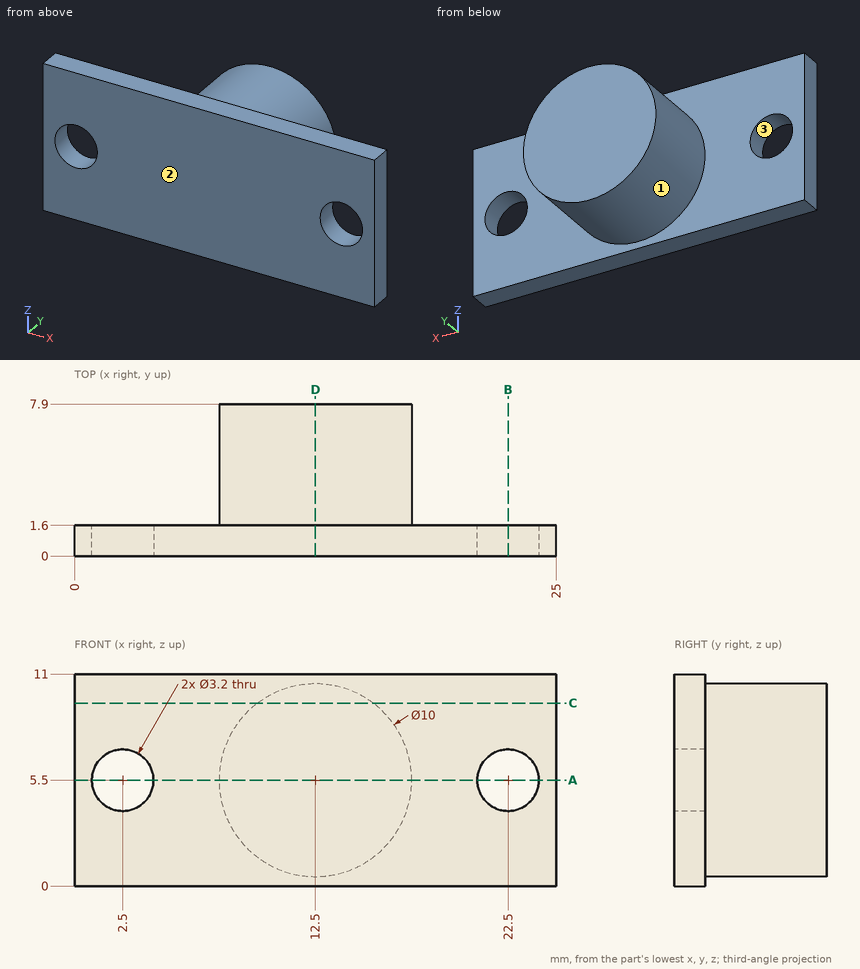
Drawing for the job (mm, zero at the part's lowest x, y, z). Give positions to 0.01 mm unless a question says otherwise; leave off trailing zeros. Order: outer loops, then holes, each group sorted by start corner. A loop starts at its lowest first (then second) coordinate and runs counter-clockwise, first axis right, second up. Notation, with made-up numbers: M 5.5,59 L 33.5,59 A7 ccw 33.5,65 Z; hole C 86.5,79.5 d6. An arc over 180 degrees is marked long. Put each result on its own line as item: value. Start each with the question number.
(1) Saw through at B-B, the plane x = 22.5. Write the cut outline in (y, z), then the cut area to 3 significant figures.
(2) Mould opens along X. For the marked faces 1, 2 and 3 say: +X half, -X half, draft (parallel to the pull), parting line (faces both ways), or undercut.
(3) Flat gauge pins, fed straight in: pin 1 Ø2.5 at (x, z) = (22.5, 5.5) entering from +Y; pin 2 Ø3.5 at (x, z) = (2.5, 5.5) entering from +Y; pin 3 Ø1.5 at (x, y) = (13.5, 6) entering from +Z. Where does each tip first touch, or does it go through?
(4) Saw through at D-D, the plane x = 12.5. Write the cut outline in (y, z), then the cut area to 3 significant figures.
(5) Drill centre lines: line 1 along X through (y, z) = (1.35, 5.5); line 2 along Z through (x, y) = (2.5, 0.85); line 3 along Y through (x, z) = (20, 4.5). Where is each one in solid material? Low to high.
(6) Saw through at C-C, the plane z = 9.5. Write the cut outline in (x, y).
(7) Saw through at A-A, the plane z = 5.5. Write the cut outline in (x, y), then the cut area to 3 significant figures.
Check result:
1. outline: M 0,0 L 1.6,0 L 1.6,3.9 L 0,3.9 Z; M 0,7.1 L 1.6,7.1 L 1.6,11 L 0,11 Z
1. area: 12.5 mm2
2. face 1: parting line
2. face 2: draft
2. face 3: undercut
3. pin 1: passes through
3. pin 2: stops at y = 1.6
3. pin 3: stops at z = 10.49
4. outline: M 0,0 L 1.6,0 L 1.6,0.5 L 7.9,0.5 L 7.9,10.5 L 1.6,10.5 L 1.6,11 L 0,11 Z
4. area: 80.6 mm2
5. line 1: x = 0 to 0.9, 4.1 to 20.9, 24.1 to 25
5. line 2: z = 0 to 3.9, 7.1 to 11
5. line 3: y = 0 to 1.6
6. outline: M 0,0 L 25,0 L 25,1.6 L 15.5,1.6 L 15.5,7.9 L 9.5,7.9 L 9.5,1.6 L 0,1.6 Z
7. outline: M 0,0 L 0.9,0 L 0.9,1.6 L 0,1.6 Z; M 4.1,0 L 20.9,0 L 20.9,1.6 L 17.5,1.6 L 17.5,7.9 L 7.5,7.9 L 7.5,1.6 L 4.1,1.6 Z; M 24.1,0 L 25,0 L 25,1.6 L 24.1,1.6 Z
7. area: 92.8 mm2
